from build123d import *

# Parameters (mm, degrees)
CROQUIS4_R            = 19
CORTAR_EXTRUIR1_DEPTH = 5
CHAFL_N1_SIZE         = 1
CHAFL_N2_SIZE         = 0.5
CHAFL_N3_SIZE         = 1
CROQUIS5_R            = 1.25
CORTAR_EXTRUIR2_DEPTH = 7.5
CHAFL_N4_SIZE         = 0.2


with BuildPart() as part:
    # Croquis1 → Revolución2 (revolve)
    with BuildSketch(Plane(origin=(0, 0, 0), x_dir=(0, 0, -1), z_dir=(1, 0, 0)), mode=Mode.PRIVATE) as revoluci_n2_sk:
        Polygon((-5.505325444, 0), (7.594674556, 0), (7.594674556, 7), (-6.505325444, 7), (-7.505325444, 6), (-7.505325444, 2), align=None)
    revolve(revoluci_n2_sk.sketch.rotate(Axis((0, -18, -7.594674556), (0, 0, 1)), 90), axis=Axis((0, -18, -7.594674556), (0, 0, 1)))

    # Croquis4 → Cortar-Extruir1 (cut)
    with BuildSketch(Plane(origin=(0, 0, -7.594674556), x_dir=(-1, 0, 0), z_dir=(0, 0, -1))):
        with Locations((0, -18)):
            Circle(CROQUIS4_R)
    extrude(amount=-CORTAR_EXTRUIR1_DEPTH, mode=Mode.SUBTRACT)

    # Chaflán1
    chafl_n1_edges = [part.edges().sort_by_distance(p)[0] for p in [
        (18, -18, -2.594674556),
    ]]
    chamfer(chafl_n1_edges, length=CHAFL_N1_SIZE - 0.0001)  # a hair under: the kernel refuses the full size

    # Chaflán2
    chafl_n2_edges = [part.edges().sort_by_distance(p)[0] for p in [
        (25, -18, -7.594674556),
    ]]
    chamfer(chafl_n2_edges, length=CHAFL_N2_SIZE)

    # Chaflán3
    chafl_n3_edges = [part.edges().sort_by_distance(p)[0] for p in [
        (19, -18, -7.594674556),
    ]]
    chamfer(chafl_n3_edges, length=CHAFL_N3_SIZE)

    # Croquis5 → Cortar-Extruir2 (cut)
    with BuildSketch(Plane(origin=(0, 0, -7.594674556), x_dir=(-1, 0, 0), z_dir=(0, 0, -1))):
        with Locations((0, 4)):
            Circle(CROQUIS5_R)
        with Locations((11, 1.052558883)):
            Circle(CROQUIS5_R)
        with Locations((19.052558883, -7)):
            Circle(CROQUIS5_R)
        with Locations((22, -18)):
            Circle(CROQUIS5_R)
        with Locations((19.052558883, -29)):
            Circle(CROQUIS5_R)
        with Locations((11, -37.052558883)):
            Circle(CROQUIS5_R)
        with Locations((0, -40)):
            Circle(CROQUIS5_R)
        with Locations((-11, -37.052558883)):
            Circle(CROQUIS5_R)
        with Locations((-19.052558883, -29)):
            Circle(CROQUIS5_R)
        with Locations((-22, -18)):
            Circle(CROQUIS5_R)
        with Locations((-19.052558883, -7)):
            Circle(CROQUIS5_R)
        with Locations((-11, 1.052558883)):
            Circle(CROQUIS5_R)
    extrude(amount=-CORTAR_EXTRUIR2_DEPTH, mode=Mode.SUBTRACT)

    # Chaflán4
    chafl_n4_edges = [part.edges().sort_by_distance(p)[0] for p in [
        (1.25, 4, -7.594674556),
        (12.25, 1.052558883, -7.594674556),
        (20.302558883, -7, -7.594674556),
        (23.25, -18, -7.594674556),
        (-9.75, 1.052558883, -7.594674556),
        (-17.802558883, -7, -7.594674556),
        (-20.75, -18, -7.594674556),
        (-17.802558883, -29, -7.594674556),
        (-9.75, -37.052558883, -7.594674556),
        (1.25, -40, -7.594674556),
        (12.25, -37.052558883, -7.594674556),
        (20.302558883, -29, -7.594674556),
    ]]
    chamfer(chafl_n4_edges, length=CHAFL_N4_SIZE)


solid = part.part
Build history of the part. All positions in model axes, mm. Round coordinates to 2 decimals unless told otherwise and drop trailing zeros. One line per item, written item: value. Start each with the question number.
Q1. Probe line 1 along X through (y, z) = (-17, -6.5); line 2 along Y through (x, z) = (0, -4.5); line 3 along X through (y, z) = (-13.5, -6.5). List the from-to ranges inside material, lowest first.
Q2. Two-plate mould, pull along Y, no slides. Class faces 1 (the face through (-11, -37, -0.095)), 2 (the face through (-11.5, 4.2, -0.2)): released by +Y, released by -Y, zero draft, split by the parting line, or undercut.
Q3. Drop flat-ended pins along their axis: pin 1 Ø3 at (y, z) = (-12, 3.5) entering from -X; pin 2 Ø1.2 at (x, y) = (-10.5, -37) entering from -Z; pin 3 Ø1 at (x, z) = (-11, -5.5) entering from -Y. Give the stop position or say it passes through.
Computed:
1. line 1: -24.98 to -22.75, -21.25 to -18.97, 18.97 to 21.25, 22.75 to 24.98
1. line 2: -43 to -41.25, -38.75 to -37, 1 to 2.75, 5.25 to 7
1. line 3: -24.59 to -18.46, 18.46 to 24.59
2. face 1: undercut
2. face 2: split by the parting line
3. pin 1: x = -24.59
3. pin 2: z = -0.09
3. pin 3: y = -40.69
